from build123d import *

# Parameters (mm, degrees)
SKETCH2_W           = 68.58
SKETCH2_H           = 24.13
SKETCH2_R           = 2.6
BOSS_EXTRUDE1_DEPTH = 6.35
CUT_EXTRUDE1_DEPTH  = 7.35
FILLET3_R           = 2.54
SKETCH4_R           = 2.5
CUT_EXTRUDE2_DEPTH  = 7.3500001


with BuildPart() as part:
    # Sketch2 → Boss-Extrude1 (new body)
    with BuildSketch(Plane(origin=(0, 0, 0), x_dir=(1, 0, 0), z_dir=(0, 1, 0))):
        with Locations((34.29, 12.065)):
            Rectangle(SKETCH2_W, SKETCH2_H)
        with Locations((4.57, 12.065)):
            Circle(SKETCH2_R, mode=Mode.SUBTRACT)
        with Locations((64.01, 12.065)):
            Circle(SKETCH2_R, mode=Mode.SUBTRACT)
    extrude(amount=BOSS_EXTRUDE1_DEPTH)

    # Sketch3 → Cut-Extrude1 (cut, through all)
    with BuildSketch(Plane(origin=(0, 6.35, 0), x_dir=(1, 0, 0), z_dir=(0, 1, 0))):
        with BuildLine():
            Line((4.57, 3.715), (0, 3.715))
            Line((0, 3.715), (0, 0))
            Line((0, 0), (6.57, 0))
            Line((6.57, 0), (6.57, 1.715))
            ThreePointArc((6.57, 1.715), (5.984213562, 3.129213562), (4.57, 3.715))
        make_face()
        with BuildLine():
            ThreePointArc((4.57, 20.415), (5.984213562, 21.000786438), (6.57, 22.415))
            Line((6.57, 22.415), (6.57, 24.13))
            Line((6.57, 24.13), (0, 24.13))
            Line((0, 24.13), (0, 20.415))
            Line((0, 20.415), (4.57, 20.415))
        make_face()
    extrude(amount=-CUT_EXTRUDE1_DEPTH, mode=Mode.SUBTRACT)

    # Fillet3
    fillet3_edges = [part.edges().sort_by_distance(p)[0] for p in [
        (6.57, 3.175, 0),
        (0, 3.175, -3.715),
        (0, 3.175, -20.415),
        (6.57, 3.175, -24.13),
    ]]
    fillet(fillet3_edges, radius=FILLET3_R)

    # Sketch4 → Cut-Extrude2 (cut, through all)
    with BuildSketch(Plane(origin=(0, 6.35, 0), x_dir=(1, 0, 0), z_dir=(0, 1, 0))):
        with Locations((34.29, 12.065)):
            Circle(SKETCH4_R)
    extrude(amount=-CUT_EXTRUDE2_DEPTH, mode=Mode.SUBTRACT)

    # Sketch8 one side → Cut-Revolve6 (revolve, cut)
    with BuildSketch(Plane(origin=(34.29, 0, 0), x_dir=(0, 0, -1), z_dir=(1, 0, 0))):
        with BuildLine():
            Line((12.065, 0), (22.13, 0))
            ThreePointArc((22.13, 0), (17.5473974, 3.215969501), (12.065, 4.35))
            Line((12.065, 4.35), (12.065, 0))
        make_face()
    revolve(axis=Axis((34.29, 6.35, -12.065), (0, -1, 0)), mode=Mode.SUBTRACT)


solid = part.part
The listing builds one solid part. Answer for the finished solid, in the listing's coordinates (mm). A direction names the side the tool comes from. Give positions to 0.01 mm unless a question says otherwise; leave off trailing zeros. Loops run counter-clockwise (first coordinate to the right, second up) from the corner with the lowest first, then second, coordinate; pieces in that order, holes last.
Item 1: Each of these flat-tipped pins is pushed along its axis until it touches: pin 1 Ø1 at (x, y) = (4, 3) entering from -Z (3 decimals); pin 2 Ø0.6 at (x, y) = (3.5, 2.5) entering from +Z (3 decimals); pin 3 Ø2 at (x, z) = (36.5, -7) entering from -Y. Where does it stop, or does it pass through?
Derived:
pin 1: stops at z = -20.415
pin 2: stops at z = -3.715
pin 3: stops at y = 2.71
Item 2: A cutting plane is placed at A-A (x = 34.29). Give the vertices of the cut face in (y, z) (3 decimals).
Derived:
outline: (0, -24.13) - (6.35, -24.13) - (6.35, -14.565) - (4.122, -14.565) arc R13.819 cw to (0, -22.13) - close; (0, -2) arc R13.819 cw to (4.122, -9.565) - (6.35, -9.565) - (6.35, 0) - (0, 0) - close
Item 3: A tool of negligible diameter and unlimited length cuts with its end or side. For faces 4 (the flat face through (4, 3, -3.715)), 5 (the flat face through (34, 0, -23)), 6 (the flat face through (4, 3, -20.415)), from which of +Z, -Z, +X, -X, +Y, -Y can it reach the whole face along a straight path? Write none if from no direction.
Derived:
face 4: +Z, -X, +Y, -Y
face 5: +Z, -Z, +X, -X, -Y
face 6: -Z, -X, +Y, -Y
Item 4: Find the intervals of material crossed by line 1 along Z through (x, y) = (34.29, 5.7) (3 decimals); line 2 along Z through (x, y) = (4.57, 4.25) (3 decimals); line 3 along X through (y, z) = (4.75, -12.25), in increasing order.
Derived:
line 1: z = -24.13 to -14.565, -9.565 to 0
line 2: z = -20.415 to -14.665, -9.465 to -3.715
line 3: x = 0 to 1.98, 7.16 to 31.8, 36.78 to 61.42, 66.6 to 68.58
Item 5: A cutting plane is placed at C-C (x = 64.01). Give the vertices of the cut face in (y, z) (3 decimals).
Derived:
outline: (0, -24.13) - (6.35, -24.13) - (6.35, -14.665) - (0, -14.665) - close; (0, -9.465) - (6.35, -9.465) - (6.35, 0) - (0, 0) - close
Item 6: A cutting plane is placed at D-D (x = 42). Give the vertices of the cut face in (y, z) (3 decimals), then the cut area to 3 significant figures.
Derived:
outline: (0, -24.13) - (6.35, -24.13) - (6.35, 0) - (0, 0) - (0, -5.595) arc R11.468 cw to (0, -18.535) - close
area: 136 mm2
Item 7: Determine the mould class of faces 1 (the flat face through (38, 3, -24.13)), 2 (the cylindrical face through (65.408, 3.131, -14.257)), 3 (the flat face through (0, 3, -12)) for opening direction X: +X half, -X half, draft (parallel to the pull), parting line (faces both ways), or undercut.
Derived:
face 1: draft
face 2: undercut
face 3: -X half
Item 8: A cutting plane is placed at B-B (z = -13.25). Give the vertices of the cut face in (x, y) (3 decimals), then the cut area to 3 significant figures.
Derived:
outline: (0, 0) - (2.256, 0) - (2.256, 6.35) - (0, 6.35) - close; (6.884, 0) - (24.295, 0) arc R13.768 cw to (32.089, 4.122) - (32.089, 6.35) - (6.884, 6.35) - close; (36.491, 4.122) arc R13.768 cw to (44.285, 0) - (61.696, 0) - (61.696, 6.35) - (36.491, 6.35) - close; (66.324, 0) - (68.58, 0) - (68.58, 6.35) - (66.324, 6.35) - close
area: 308 mm2
